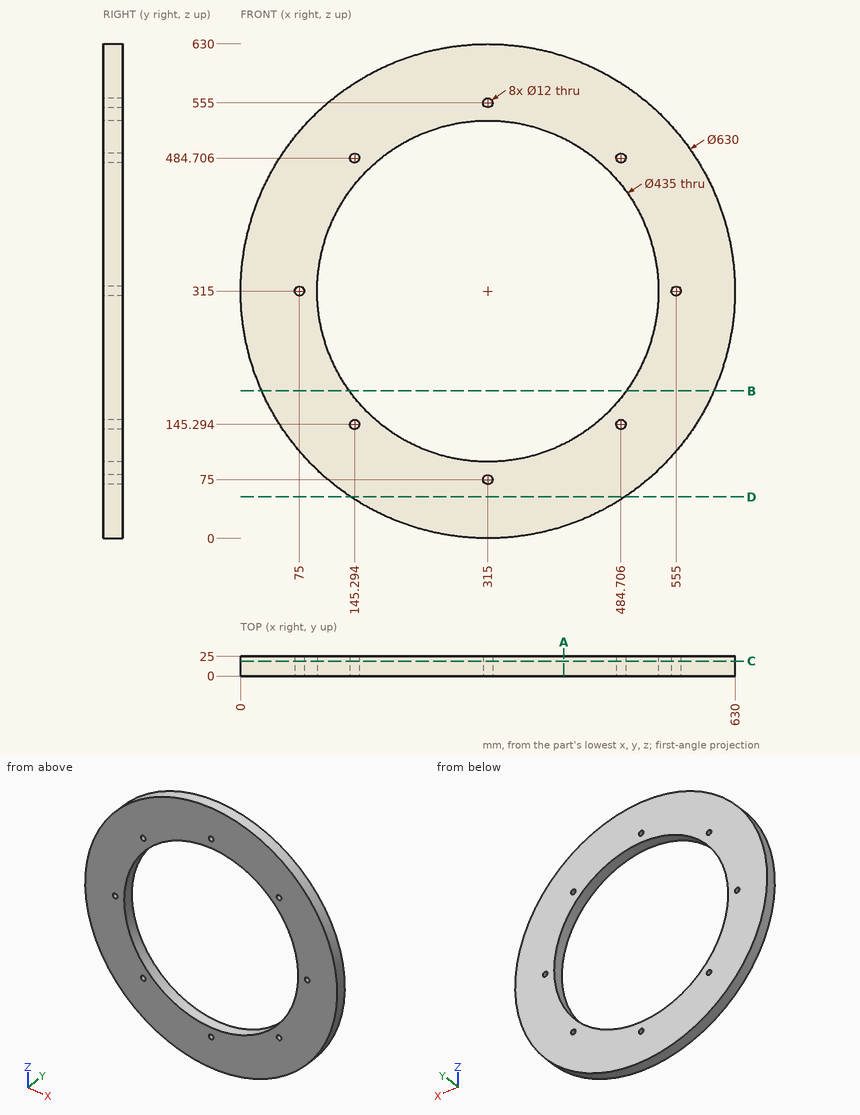
Here's the drawing with two shaded views (mm, measured from the low corner). I have some questions. Coordinates: 2 decimals unless noted, no trailing zeros. Order: outer loops, then holes, each group sorted by start corner. A loop starts at its lowest first (then second) coordinate and runs counter-clockwise, first axis right, second up. Notation, with made-up numbers: M 80,-7.5 L 133,-7.5 A19 cw 133,8.5 Z; hole C -14.5,27 d2. An arc over 180 degrees is marked long. Answer as CSV lines item,"result".
Item 1: For pin 1 (8 mm diameter, centred on y = 4, z = 229.5, fed in from +X); pin 2 (12 mm diameter, centred on x = 363, y = 7.5, fed in from -Z); pin 3 (8 mm diameter, centred on x = 72, y = 14.5, fed in from -Z), each with a flat end and sliding along its axis, tell me the tip position at first contact or that it passes through.
Results found:
pin 1,"x = 619.27"
pin 2,"z = 2.81"
pin 3,"z = 109.81"
Item 2: If I drill on line 1 (Z direction, x = 488.5, y = 18.5) (1 decimal); line 2 (X direction, y = 19, z = 498) (1 decimal); line 3 (X direction, y = 19.5, z = 286), over which ranges is the centre line in solid material (lowest first)?
Results found:
line 1,"52.1 to 140.6, 149.9 to 183.8, 446.2 to 480.1, 489.4 to 577.9"
line 2,"58.6 to 197.5, 432.5 to 571.4"
line 3,"1.34 to 99.44, 530.56 to 628.66"
Item 3: Imagine slicing it at D-D on z = 53. Write out the boundary of the cut face in (x, y).
Results found:
outline,"M 140.13,0 L 489.87,0 L 489.87,25 L 140.13,25 Z"
Item 4: Imagine slicing it at A-A on x = 412. Write out the boundary of the cut face in (y, z), plus the area to 3 significant figures.
Results found:
outline,"M 0,15.31 L 25,15.31 L 25,120.33 L 0,120.33 Z; M 0,509.67 L 25,509.67 L 25,614.69 L 0,614.69 Z"
area,"5,250 mm2"
Item 5: Imagine slicing it at B-B on z = 188. Write out the boundary of the cut face in (x, y).
Results found:
outline,"M 26.74,0 L 138.43,0 L 138.43,25 L 26.74,25 Z; M 491.57,0 L 603.26,0 L 603.26,25 L 491.57,25 Z"
Item 6: Imagine slicing it at C-C on y = 19. Give the number of separate pieces and of enclosed holes in the cut face, plus the area to 3 significant figures.
Results found:
separate pieces,"1"
enclosed holes,"9"
area,"162,000 mm2"
